The listing builds one solid part. Answer for the finished solid, in the listing's coordinates (mm). Face numbers are marked on the shaded views. A direction names the side the tool comes from. Round coordinates to 2 decimals unless told otherwise and drop trailing zeros. Write each loop counter-clockwise with the first axis right and the second up, starting at its lowest first coordinate (ties: lowest second). Pieces come first, ordered by that corner, then holes. Notation, with made-up numbers: (-14, -7.5) - (40, -7.5) arc R32 cw to (40, 30.5) - close; hole circle Ø2 at (-39.5, 20.5). An arc over 180 degrees is marked (long way). Answer as CSV lines item,"result". Start each with the question number.
Item 1: A cutting plane is placed at A-A on y = -1. Determine the outline of the cut face in (x, z).
Item 2: Flat-ended cylindrical pins translate along their axes: pin 1 (2 mm diameter, centred on x = 42, z = 2, fed in from +Y); pin 2 (1.4 mm diameter, centred on y = 0, z = -1, fed in from +X); pin 3 (1.2 mm diameter, centred on x = 57.5, z = 0, fed in from +Y). Find the tip coordinate at first contact, or state that the pin passes through.
Item 3: Which of the six approach directions +Z, -Z, +X, -X, +Y, -Y give full straight-line access (tool end or side, diameter ignored) to the marked faces 4, 5 and 6?
Item 4: A cutting plane is placed at C-C on x = 5.5. Determine the outline of the cut face in (y, z), and give its area (3 significant figures).
Item 5: Straight lines are drawn through the part: line 1 along X through (y, z) = (-0.75, 0); line 2 along Z through (x, y) = (35.5, -1.25); line 3 along X through (y, z) = (1, -3.5). For each, find the intervals that lie inside material, in ascending order. Write a range as [from, to].
Item 6: For a pull along X with two mould halves and no side action, classify the marked faces 1, 2 and 3 as pulls with the +X half, pulls with the -X half, needs draft (parallel to the pull), parting line crosses it, or undercut.
Item 7: A cutting plane is placed at B-B on x = 51. Determine the outline of the cut face in (y, z).
```python
from build123d import *

# Parameters (mm, degrees)
F0_R      = 4.086054
F1_DEPTH  = 10
F2_R      = 3.46296
F3_DEPTH  = 10
F4_R      = 2.947818
F5_DEPTH  = 10
F6_R      = 2.396376
F7_DEPTH  = 10
F8_R      = 1.894125
F9_DEPTH  = 15
F10_R     = 2.032934
F11_DEPTH = 1.5
F13_DEPTH = 12.5


with BuildPart() as f1:
    # F0 (on Right) → F1 (new body)
    with BuildSketch(Plane.YZ):
        Circle(F0_R)
    extrude(amount=F1_DEPTH)

    # F2 (on face) → F3 (join)
    with BuildSketch(Plane.YZ.offset(10)):
        Circle(F2_R)
    extrude(amount=F3_DEPTH)

    # F4 (on face) → F5 (join)
    with BuildSketch(Plane.YZ.offset(20)):
        Circle(F4_R)
    extrude(amount=F5_DEPTH)

    # F6 (on face) → F7 (join)
    with BuildSketch(Plane.YZ.offset(30)):
        Circle(F6_R)
    extrude(amount=F7_DEPTH)

    # F8 (on face) → F9 (join)
    with BuildSketch(Plane.YZ.offset(40)):
        Circle(F8_R)
    extrude(amount=F9_DEPTH)

    # F10 (on Front) → F11 (join, symmetric)
    with BuildSketch(Plane.XZ):
        with Locations((57.003621, 0)):
            Circle(F10_R)
    extrude(amount=F11_DEPTH, both=True)

    # F12 (on Front) → F13 (cut, symmetric)
    with BuildSketch(Plane.XZ):
        with BuildLine():
            ThreePointArc((7.348375, 1.011325), (6.33705, 0), (7.348375, -1.011325))
            ThreePointArc((7.348375, -1.011325), (8.3597, 0), (7.348375, 1.011325))
        make_face()
    extrude(amount=F13_DEPTH, both=True, mode=Mode.SUBTRACT)


solid = f1.part
```
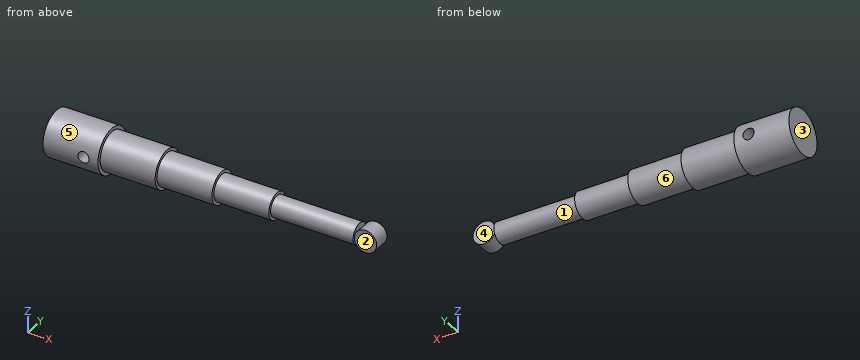
Geometry says:
1,outline,"(0, -3.96) - (10, -3.96) - (10, -3.32) - (20, -3.32) - (20, -2.77) - (30, -2.77) - (30, -2.18) - (40, -2.18) - (40, -1.61) - (55, -1.61) - (55, -0.34) arc R2.03 ccw (long way) to (55, 0.34) - (55, 1.61) - (40, 1.61) - (40, 2.18) - (30, 2.18) - (30, 2.77) - (20, 2.77) - (20, 3.32) - (10, 3.32) - (10, 3.96) - (0, 3.96) - close; hole circle Ø2.02 at (7.35, 0)"
2,pin 1,"stops at y = 1.61"
2,pin 2,"stops at x = 59.01"
2,pin 3,"stops at y = 1.5"
3,face 4,"+Z, -Z, +X, +Y"
3,face 5,"+X, -X"
3,face 6,"+X"
4,outline,"circle Ø8.17 at (0, 0)"
4,area,"52.5 mm^2"
5,line 1,"x = [0, 6.34], [8.36, 59.04]"
5,line 2,"z = [-2.04, 2.04]"
5,line 3,"x = [0, 10]"
6,face 1,"undercut"
6,face 2,"needs draft"
6,face 3,"pulls with the -X half"
7,outline,"circle Ø3.79 at (0, 0)"
